The listing builds one solid part. Answer for the finished solid, in the listing's coordinates (mm). Coordinates: 2 decimals unless noted, no trailing zeros. Loops run counter-clockwise (first coordinate to the right, second up) from the corner with the lowest first, then second, coordinate; pieces in that order, holes last. Notation, with made-up numbers: M -8,-14 L 7,-14 A9 cw 7,-9 Z; hole C 85.25,70 d1. An arc over 180 degrees is marked long. Answer as a JSON object with one key per item and string values. Group by question number.
1. Given pin 1 (14.5 mm diameter, centred on x = 0, y = -58.95, fed in from -Z); pin 2 (2 mm diameter, centred on x = -32, z = 3.5, fed in from +Y); pin 3 (2 mm diameter, centred on y = 16, z = 1.5, fed in from -X); pin 4 (2 mm diameter, centred on y = -50, z = 4.5, fed in from -X), each flat-ended and moving along its own axis, determine where each tip first touches the part or whether it passes through.
2. A cutting plane is placed at A-A on z = 2. State how many separate pieces and enclosed holes the cut face has, and give its area (3 significant figures).
3. Determine the mould class of faces 1 (the face through (-9.373, 71.387, 3.131)), 2 (the face through (-1, -15, 0)), 3 (the face through (66.604, 2.41, 3.131)) for opening direction Y: released by +Y, released by -Y, zero draft, split by the parting line, or undercut.
4. A cutting plane is placed at B-B on y = 63.5. Give the vertices of the cut face in (x, z), and give its area (3 significant figures).
5. A cutting plane is placed at C-C on x = 54.5. Give the vertices of the cut face in (y, z).
6. A cutting plane is placed at D-D on x = 25. Give the vertices of the cut face in (y, z), and give its area (3 significant figures).
7. Straight lines are drawn through the part: L1, parallel to Y at x = 0, z = 2.75 (3 decimals); L2, parallel to Y at x = -57.5, z = 4.5; L3, parallel to X at y = -47, z = 0.75. For each, find the intervals that lie inside material, in ascending order.
from build123d import *

# Parameters (mm, degrees)
SKETCH1_R             = 72
SKETCH1_R_2           = 8.025
BOSS_EXTRUDE1_DEPTH   = 6.35
SKETCH2_R             = 2.5
CUT_EXTRUDE1_DEPTH    = 10
M3X0_5_TAPPED_HOLE1_D = 2.5
M3X0_5_TAPPED_HOLE2_D = 2.5
M3X0_5_TAPPED_HOLE3_D = 2.5
M3X0_5_TAPPED_HOLE4_D = 2.5


with BuildPart() as part:
    # Sketch1 → Boss-Extrude1 (new body)
    with BuildSketch(Plane.XY):
        Circle(SKETCH1_R)
        with Locations((58.95, 0)):
            Circle(SKETCH1_R_2, mode=Mode.SUBTRACT)
        with Locations((51.052197553, 29.475)):
            Circle(SKETCH1_R_2, mode=Mode.SUBTRACT)
        with Locations((29.475, 51.052197553)):
            Circle(SKETCH1_R_2, mode=Mode.SUBTRACT)
        with Locations((0, 58.95)):
            Circle(SKETCH1_R_2, mode=Mode.SUBTRACT)
        with Locations((-29.475, 51.052197553)):
            Circle(SKETCH1_R_2, mode=Mode.SUBTRACT)
        with Locations((-51.052197553, 29.475)):
            Circle(SKETCH1_R_2, mode=Mode.SUBTRACT)
        with Locations((-58.95, 0)):
            Circle(SKETCH1_R_2, mode=Mode.SUBTRACT)
        with Locations((-51.052197553, -29.475)):
            Circle(SKETCH1_R_2, mode=Mode.SUBTRACT)
        with Locations((-29.475, -51.052197553)):
            Circle(SKETCH1_R_2, mode=Mode.SUBTRACT)
        with Locations((0, -58.95)):
            Circle(SKETCH1_R_2, mode=Mode.SUBTRACT)
        with Locations((29.475, -51.052197553)):
            Circle(SKETCH1_R_2, mode=Mode.SUBTRACT)
        with Locations((51.052197553, -29.475)):
            Circle(SKETCH1_R_2, mode=Mode.SUBTRACT)
    extrude(amount=BOSS_EXTRUDE1_DEPTH)

    # Sketch2 → Cut-Extrude1 (cut)
    with BuildSketch(Plane.XY.offset(6.35)):
        Circle(SKETCH2_R)
    extrude(amount=-CUT_EXTRUDE1_DEPTH, mode=Mode.SUBTRACT)

    # M3x0.5 Tapped Hole1 (through all)
    with Locations(Plane(origin=(-6.94699298, 0, 6.35), x_dir=(1, 0, 0), z_dir=(0, 0, 1))):
        with Locations((0, 0)):
            Hole(M3X0_5_TAPPED_HOLE1_D / 2)

    # M3x0.5 Tapped Hole2 (through all)
    with Locations(Plane(origin=(0, 7, 6.35), x_dir=(1, 0, 0), z_dir=(0, 0, 1))):
        with Locations((0, 0)):
            Hole(M3X0_5_TAPPED_HOLE2_D / 2)

    # M3x0.5 Tapped Hole3 (through all)
    with Locations(Plane(origin=(0, -7, 6.35), x_dir=(1, 0, 0), z_dir=(0, 0, 1))):
        with Locations((0, 0)):
            Hole(M3X0_5_TAPPED_HOLE3_D / 2)

    # M3x0.5 Tapped Hole4 (through all)
    with Locations(Plane(origin=(7, 0, 6.35), x_dir=(1, 0, 0), z_dir=(0, 0, 1))):
        with Locations((0, 0)):
            Hole(M3X0_5_TAPPED_HOLE4_D / 2)


solid = part.part
From the geometry:
{
 "1": {"pin 1": "passes through", "pin 2": "stops at y = 64.98", "pin 3": "stops at x = -70.42", "pin 4": "stops at x = -52.75"},
 "2": {"separate pieces": "1", "enclosed holes": "17", "area": "13,800 mm²"},
 "3": {"face 1": "split by the parting line", "face 2": "zero draft", "face 3": "undercut"},
 "4": {"outline": "M -33.94,0 L -6.61,0 L -6.61,6.35 L -33.94,6.35 Z; M 6.61,0 L 33.94,0 L 33.94,6.35 L 6.61,6.35 Z", "area": "347 mm²"},
 "5": {"outline": "M -47.05,0 L -36.72,0 L -36.72,6.35 L -47.05,6.35 Z; M -22.23,0 L -6.68,0 L -6.68,6.35 L -22.23,6.35 Z; M 6.68,0 L 22.23,0 L 22.23,6.35 L 6.68,6.35 Z; M 36.72,0 L 47.05,0 L 47.05,6.35 L 36.72,6.35 Z"},
 "6": {"outline": "M -67.52,0 L -57.71,0 L -57.71,6.35 L -67.52,6.35 Z; M -44.39,0 L 44.39,0 L 44.39,6.35 L -44.39,6.35 Z; M 57.71,0 L 67.52,0 L 67.52,6.35 L 57.71,6.35 Z", "area": "688 mm²"},
 "7": {"L1": "y = -72 to -66.975, -50.925 to -8.25, -5.75 to -2.5, 2.5 to 5.75, 8.25 to 50.925, 66.975 to 72", "L2": "y = -43.33 to -34.25, -24.7 to -7.89, 7.89 to 24.7, 34.25 to 43.33", "L3": "x = -54.54 to -36.4, -22.55 to 22.55, 36.4 to 54.54"}
}
